Model file for the job. Use its own axes, mm. A direction names the side the tool comes from. Coordinates: 2 decimals unless noted, no trailing zeros. Order: outer loops, then holes, each group sorted by start corner. A loop starts at its lowest first (then second) coordinate and runs counter-clockwise, first axis right, second up. Notation, with made-up numbers: (17, 59.25) -> (28, 59.25) arc R23 cw to (28, 76.25) -> close; hole circle Ø10 at (-31.75, 38.25). An arc over 180 degrees is marked (long way). Return JSON: item names as keys, results as strings. Group by question number.
1) Cut at A-A (y = -28). Write the cut outline in (x, z) (3 decimals).
2) Cut at B-B (z = 16). Write the cut outline in (x, y) (3 decimals).
3) Flat gauge pins, fed straight in: pin 1 (3 mm diameter, centred on x = -21, y = 15.5, fed in from +Z); pin 2 (1.5 mm diameter, centred on x = 5.5, z = 14.5, fed in from -Y). Where does each tip first touch, or does it go through?
4) Cut at D-D (x = 9). Write the cut outline in (y, z).
5) Which spindle directions (+Z, -Z, +X, -X, +Y, -Y) get a long thin tool onto all of the face, cutting with end or side? Do faces 1 (the flat face through (0, 5, 22)), 2 (the flat face through (20.36, 19.42, 22.18)), 3 (the flat face through (21, 22, 22)), 4 (the cylindrical face through (25.07, 20.5, 22.82)), 5 (the flat face through (0, 0, 22)). Say none if no direction does.
6) Probe line 1 (X direction, y = -27, z = 23) (3 decimals); line 2 (X direction, y = 14, z = 20); line 3 (Y direction, x = -4.5, z = 3.5). List the from-to ranges inside material, lowest first.
7) Pull direction X, two halves, no side cores. Call faces 6 (the flat face through (4, 2, 0)), 7 (the cylindrical face through (-25, 20.57, 22.82)), 8 (the flat face through (20.155, -20, 22)): +X half, -X half, draft (parallel to the pull), parting line (faces both ways), or undercut.
8) Cut at C-C (y = 7). Write the cut outline in (x, z).
from build123d import *

# Parameters (mm, degrees)
F1_DEPTH = 45
F2_R     = 5
F3_R     = 5
F4_R     = 5


with BuildPart() as f1:
    # F0 (on Top) → F1 (new body)
    with BuildSketch(Plane.XY):
        Polygon((-26.5, -35), (-20.155, -35), (-20.155, 0), (20.155, 0), (20.155, -35), (26.5, -35), (26.5, 22), (21.5, 22), (19.5, 22), (21.5, 16), (21.5, 5), (-21.5, 5), (-21.5, 16), (-19.5, 22), (-21.5, 22), (-26.5, 22), align=None)
    extrude(amount=F1_DEPTH)

    # F2
    f2_edges = [f1.edges().sort_by_distance(p)[0] for p in [
        (26.5, -35, 22.5),
        (-26.5, -35, 22.5),
        (-26.5, 22, 22.5),
        (26.5, 22, 22.5),
    ]]
    fillet(f2_edges, radius=F2_R)

    # F3
    f3_edges = [f1.edges().sort_by_distance(p)[0] for p in [
        (-21.5, 16, 22.5),
        (21.5, 16, 22.5),
        (-21.5, 5, 22.5),
        (21.5, 5, 22.5),
    ]]
    fillet(f3_edges, radius=F3_R)

    # F4
    f4_edges = [f1.edges().sort_by_distance(p)[0] for p in [
        (-20.155, 0, 22.5),
        (20.155, 0, 22.5),
    ]]
    fillet(f4_edges, radius=F4_R)


solid = f1.part
Answers below:
{
 "1": {"outline": "(-26.5, 0) -> (-20.155, 0) -> (-20.155, 45) -> (-26.5, 45) -> close; (20.155, 0) -> (26.5, 0) -> (26.5, 45) -> (20.155, 45) -> close"},
 "2": {"outline": "(-26.5, -30) arc R5 ccw to (-21.5, -35) -> (-20.155, -35) -> (-20.155, -5) arc R5 cw to (-15.155, 0) -> (15.155, 0) arc R5 cw to (20.155, -5) -> (20.155, -35) -> (21.5, -35) arc R5 ccw to (26.5, -30) -> (26.5, 17) arc R5 ccw to (21.5, 22) -> (19.5, 22) -> (21.243, 16.77) arc R5 cw to (21.5, 15.189) -> (21.5, 10) arc R5 cw to (16.5, 5) -> (-16.5, 5) arc R5 cw to (-21.5, 10) -> (-21.5, 15.189) arc R5 cw to (-21.243, 16.77) -> (-19.5, 22) -> (-21.5, 22) arc R5 ccw to (-26.5, 17) -> close"},
 "3": {"pin 1": "stops at z = 45", "pin 2": "stops at y = 0"},
 "4": {"outline": "(0, 0) -> (5, 0) -> (5, 45) -> (0, 45) -> close"},
 "5": {"face 1": "+Z, -Z, +Y", "face 2": "+Z, -Z", "face 3": "+Z, -Z, +X, -X, +Y", "face 4": "+Z, -Z, +X, +Y", "face 5": "+Z, -Z, -Y"},
 "6": {"line 1": "x = -26.5 to -20.155, 20.155 to 26.5", "line 2": "x = -26.5 to -21.5, 21.5 to 26.5", "line 3": "y = 0 to 5"},
 "7": {"face 6": "draft", "face 7": "-X half", "face 8": "undercut"},
 "8": {"outline": "(-26.5, 0) -> (-20.5, 0) -> (-20.5, 45) -> (-26.5, 45) -> close; (20.5, 0) -> (26.5, 0) -> (26.5, 45) -> (20.5, 45) -> close"}
}
